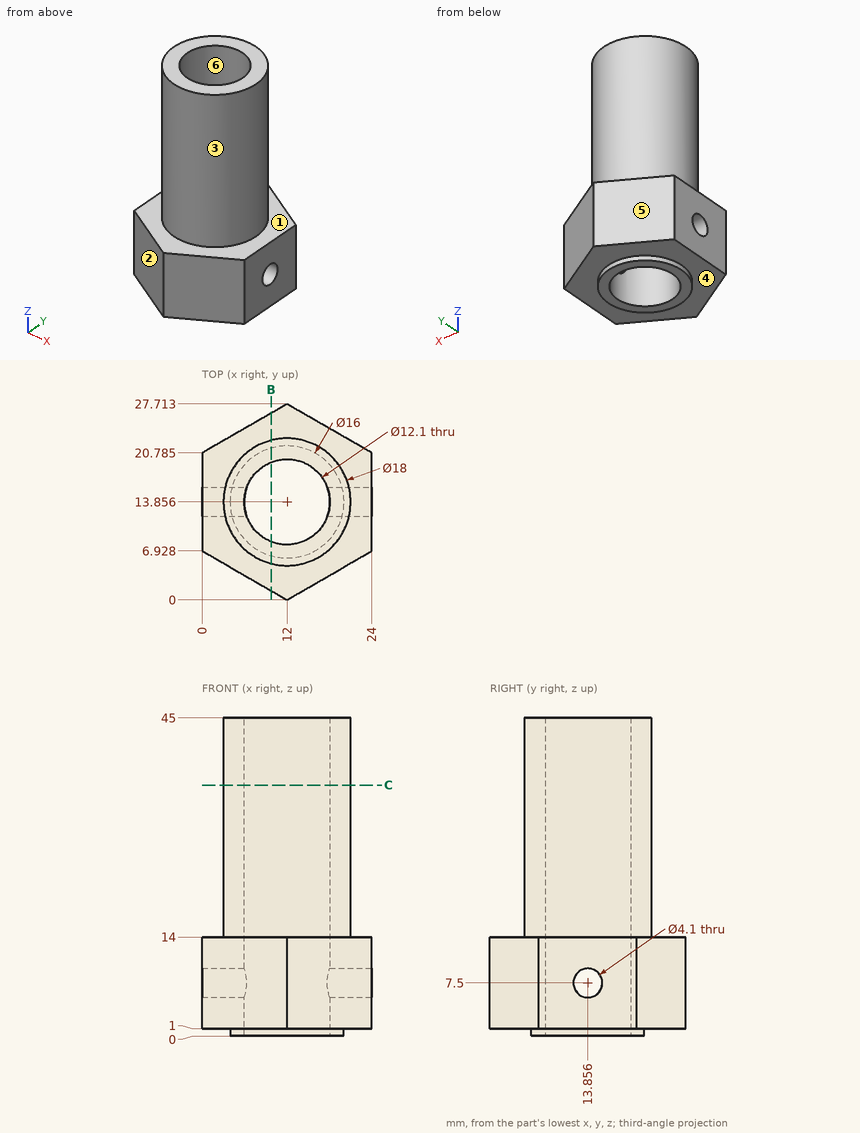
Study the drawing (mm; zero at the part's minimum x, y, z) and answer. A direction names the side the tool comes from. Coordinates: 2 decimals unless noted, no trailing zeros. Write each loop counter-clockwise with the first axis right and the second up, starting at its lowest first coordinate (ties: lowest second). Pieces come first, ordered by that corner, then holes.
Q1. Given P1, Ø6, axis at y = 13, z = 27, coming from the +X side; P2, Ø8, axis at x = 4, z = 28, coming from the +Y side; P3, Ø1, axis at x = 9.5, z = 18, coming from the -Y side; P4, Ø3.5, axis at y = 13.86, z = 7.5, coming from the +X side, each flat-ended and moving along its own axis, determine where each tip first touches the part or whether it passes through.
Returned:
P1: stops at x = 21
P2: stops at y = 21.92
P3: stops at y = 5.08
P4: passes through
Q2. Find the intervals of material crossed by line 1 along Y through (x, z) = (12.25, 36); line 2 along X through (y, z) = (14, 35.5); line 3 along Y through (x, z) = (12.75, 16) (1 decimal), in increasing order.
Returned:
line 1: y = 4.86 to 7.81, 19.9 to 22.85
line 2: x = 3 to 5.95, 18.05 to 21
line 3: y = 4.9 to 7.9, 19.9 to 22.8
Q3. Which of the six approach directions +Z, -Z, +X, -X, +Y, -Y give full straight-line access (tool end or side, diameter ignored) to the marked faces 1 and 2?
Returned:
face 1: +Z
face 2: +Z, -Z, -X, -Y
Q4. Section B-B, the plane x = 9.75 is taken. Write down the section's boundary in (y, z), then the cut area to 3 significant figures.
Returned:
outline: (1.3, 1) - (6.18, 1) - (6.18, 0) - (8.24, 0) - (8.24, 45) - (5.14, 45) - (5.14, 14) - (1.3, 14) - close; (19.47, 0) - (21.53, 0) - (21.53, 1) - (26.41, 1) - (26.41, 14) - (22.57, 14) - (22.57, 45) - (19.47, 45) - close
area: 377 mm2
Q5. The mould has two halves that part along Y. Classify the marked faces 3, 4, 5 and 6: released by +Y, released by -Y, zero draft, split by the parting line, or undercut.
Returned:
face 3: split by the parting line
face 4: zero draft
face 5: released by +Y
face 6: undercut
Q6. Section C-C, the plane z = 35.5 is taken. Write down the section's boundary in (x, y).
Returned:
outline: circle Ø18 at (12, 13.86); hole circle Ø12.1 at (12, 13.86)
